Geometry check sheet. Reference: the model listing, model coordinates, mm. Coordinates: 2 decimals unless noted, no trailing zeros. Write each loop counter-clockwise with the first axis right and the second up, starting at its lowest first coordinate (ties: lowest second). Pieces come first, ordered by that corner, then holes. Notation, with made-up numbers: M 89,-26.5 L 102,-26.5 A35 cw 102,5.5 Z; hole C 88.5,81 d9. An arc over 180 degrees is marked long. Put each result on its own line as item: value. Start each with the question number.
1) Scan lines: line 1 along X through (y, z) = (11.5, 0.25); line 2 along Z through (x, y) = (-3.5, 10.25). Record each from-to range of solid material in increasing order.
2) Cross-section at A-A on x = 0. Record the cut outline in (y, z).
3) Cross-section at B-B on z = 0. Record the cut outline in (x, y), plus the area to 3 significant figures.
4) Cross-section at C-C on y = 11.25. Record the cut outline in (x, z).
5) Gauge pin test, flat ends, axial feed: pin 1 (4 mm diameter, centred on x = -2, y = 7.5, fed in from +Z); pin 2 (3 mm diameter, centred on x = 5, y = 14, fed in from +Z); pin 3 (5.5 mm diameter, centred on x = 0.5, z = 2.5, fed in from -Y); pin 4 (2 mm diameter, centred on y = 1.5, z = 4.5, fed in from -X). Record the tip position at first contact, or that the pin passes through.
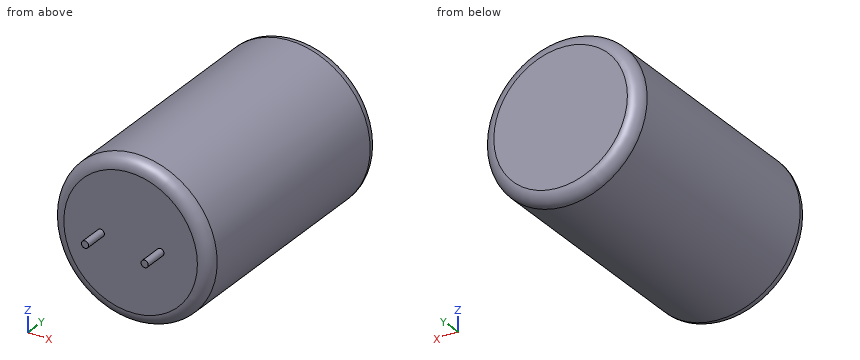
from build123d import *

# Parameters (mm, degrees)
SKETCH1_R           = 6.6
BOSS_EXTRUDE1_DEPTH = 21.4
FILLET1_R           = 1
SKETCH2_R           = 0.3
BOSS_EXTRUDE2_DEPTH = 2


with BuildPart() as part:
    # Sketch1 → Boss-Extrude1 (new body)
    with BuildSketch(Plane(origin=(0, 0, 0), x_dir=(1, 0, 0), z_dir=(0, 1, 0))):
        Circle(SKETCH1_R)
    extrude(amount=BOSS_EXTRUDE1_DEPTH)

    # Fillet1
    fillet1_edges = [part.edges().sort_by_distance(p)[0] for p in [
        (-6.6, 0, 0),
        (-6.6, 21.4, 0),
    ]]
    fillet(fillet1_edges, radius=FILLET1_R)

    # Sketch2 → Boss-Extrude2 (add)
    with BuildSketch(Plane.XZ):
        with Locations((-2.5, 0)):
            Circle(SKETCH2_R)
        with Locations((2.5, 0)):
            Circle(SKETCH2_R)
    extrude(amount=BOSS_EXTRUDE2_DEPTH)


solid = part.part
Answer key:
1. line 1: x = -6.6 to 6.6
1. line 2: z = -5.6 to 5.6
2. outline: M 0,-5.6 A1 ccw 1,-6.6 L 20.4,-6.6 A1 ccw 21.4,-5.6 L 21.4,5.6 A1 ccw 20.4,6.6 L 1,6.6 A1 ccw 0,5.6 Z
3. outline: M -6.6,1 A1 ccw -5.6,0 L -2.8,0 L -2.8,-2 L -2.2,-2 L -2.2,0 L 2.2,0 L 2.2,-2 L 2.8,-2 L 2.8,0 L 5.6,0 A1 ccw 6.6,1 L 6.6,20.4 A1 ccw 5.6,21.4 L -5.6,21.4 A1 ccw -6.6,20.4 Z
3. area: 284 mm²
4. outline: C 0,0 d13.2
5. pin 1: stops at z = 6.6
5. pin 2: stops at z = 5.6
5. pin 3: stops at y = 0
5. pin 4: stops at x = -5.6
